Autodesk Inventor part; units mm, degrees
ref_plane "YZ Plane" through (0, 0, 0) normal (1, 0, 0) x (0, 1, 0)
ref_plane "XZ Plane" through (0, 0, 0) normal (0, 1, 0) x (-1, 0, 0)
ref_plane "XY Plane" through (0, 0, 0) normal (0, 0, 1) x (1, 0, 0)
sketch "Sketch1" plane through (0, 0, 0) normal (0, 1, 0) x (-1, 0, 0)
  arc A0 (-25.4, 0) -> (25.4, 0) centre (0, 0) ccw
  arc A1 (-35.4, 0) -> (35.4, 0) centre (0, 0) ccw
  line L0 (-35.4, 0) -> (-25.4, 0)
  line L1 (25.4, 0) -> (35.4, 0)
  line L2 (35.4, 0) -> (55.4, 0)
  line L3 (55.4, 0) -> (55.4, -10)
  line L4 (55.4, -10) -> (33.9582, -10)
  line L5 (-35.4, 0) -> (-55.4, 0)
  line L6 (-55.4, 0) -> (-55.4, -10)
  line L7 (-55.4, -10) -> (-33.9582, -10)
  dimension "d0" = 50.8
  dimension "d1" = 10
  dimension "d2" = 20
  dimension "d3" = 10
  dimension "d4" = 20
  dimension "d5" = 10
extrude "Extrusion1" add sketch "Sketch1" along normal blind 40
sketch "Sketch2" plane through (-55.4, 0, 0) normal (0, 0, 1) x (1, 0, 0)
  circle A0 centre (10, 20) radius 2.75
  circle A1 centre (100.8, 20) radius 2.75
  line L0 (80.8, 40) -> (110.8, 40)
  line L1 (110.8, 0) -> (110.8, 40)
  line L2 (0, 0) -> (0, 40)
  line L3 (0, 40) -> (30, 40)
  point P0 (55.4, 0)
  dimension "d8" = 5.5
  dimension "d9" = 5.5
  dimension "d10" = 20
  dimension "d11" = 10
  dimension "d12" = 10
  dimension "d13" = 20
extrude "Extrusion2" cut sketch "Sketch2" against normal blind 40
Source: CAD feature listing. Evaluate the final solid. Frame: model axes, mm. A direction names the side the tool comes from. Round coordinates to 2 decimals unless told otherwise and drop trailing zeros. Loops run counter-clockwise (first coordinate to the right, second up) from the corner with the lowest first, then second, coordinate; pieces in that order, holes last. Notation, with made-up numbers: (29, -17.75) -> (36, -17.75) arc R18 ccw to (36, 16.25) -> close; hole circle Ø9 at (61.25, 18.25). An arc over 180 degrees is marked (long way). Answer as a JSON object with one key per item and string values. Group by question number.
Q1. Contact query for flat-ended pins moving along their axis: P1, Ø3, axis at x = -9, y = 10.5, coming from the +Z side; P2, Ø6, axis at x = -19.5, z = -4, coming from the +Y side; P3, Ø4, axis at x = 7, y = 30.5, coming from the +Z side; P4, Ø10.5, axis at x = -41, y = 16.5, coming from the -Z side. Output: stop coordinate, or through.
Q2. Access query for faces 1 (the flat face through (1, 0, -29)), 2 (the flat face through (-42, 20, -10)), 3 (the flat face through (42, 20, -10)). Directions: +Z, -Z, +X, -X, +Y, -Y. A direction counts if a zero-diameter tool reaches every point of the face in a straight line with its end or side. Return the directions, or none.
Q3. Mould query, pull axis X, two halves, no side actions, for faces 4 (the cylindrical face through (-0.637, 19.72, -35.394)), 5 (the cylindrical face through (-48.147, 20.121, -4.93)), 6 (the flat face through (55.4, 20, -5)), 7 (the flat face through (41, 20, 0)). Classes: pulls with the +X half, pulls with the -X half, needs draft (parallel to the pull), parting line crosses it, or undercut.
Q4. Section query A-A (x = 45.4). Output: boundary loops of the cut face in (y, z), plus the area to 3 significant figures.
Q5. Section query B-B (y = 20). Output: boundary loops of the cut face in (x, z).
Q6. Section query C-C (z = -16.5). Output: boundary loops of the cut face in (x, y), plus the area to 3 significant figures.
Q7. Ray query, line 1 (Y direction, x = 45.4, z = -5); line 2 (X direction, y = 18, z = -9); line 3 (Z direction, x = 35.5, y = 18). Return the intervals inside material, ascending. Write a range as from..to.
Q8. Section query D-D (y = 8). Output: boundary loops of the cut face in (x, z).
Completed:
{
 "1": {"P1": "z = -23.13", "P2": "through", "P3": "z = -23.75", "P4": "z = -10"},
 "2": {"face 1": "+Z, -Z, +X, -X, -Y", "face 2": "-Z, -X, +Y, -Y", "face 3": "-Z, +X, +Y, -Y"},
 "3": {"face 4": "parting line crosses it", "face 5": "undercut", "face 6": "pulls with the +X half", "face 7": "needs draft"},
 "4": {"outline": "(0, -10) -> (17.25, -10) -> (17.25, 0) -> (0, 0) -> close; (22.75, -10) -> (40, -10) -> (40, 0) -> (22.75, 0) -> close", "area": "345 mm²"},
 "5": {"outline": "(-55.4, -10) -> (-48.15, -10) -> (-48.15, 0) -> (-55.4, 0) -> close; (-42.65, -10) -> (-33.96, -10) arc R35.4 ccw to (33.96, -10) -> (42.65, -10) -> (42.65, 0) -> (25.4, 0) arc R25.4 cw to (-25.4, 0) -> (-42.65, 0) -> close; (48.15, -10) -> (55.4, -10) -> (55.4, 0) -> (48.15, 0) -> close"},
 "6": {"outline": "(-31.32, 0) -> (-19.31, 0) -> (-19.31, 40) -> (-31.32, 40) -> close; (19.31, 0) -> (31.32, 0) -> (31.32, 40) -> (19.31, 40) -> close", "area": "961 mm²"},
 "7": {"line 1": "0..17.25, 22.75..40", "line 2": "-55.4..-47.29, -43.51..-23.75, 23.75..43.51, 47.29..55.4", "line 3": "-10..0"},
 "8": {"outline": "(-55.4, -10) -> (-33.96, -10) arc R35.4 ccw to (33.96, -10) -> (55.4, -10) -> (55.4, 0) -> (25.4, 0) arc R25.4 cw to (-25.4, 0) -> (-55.4, 0) -> close"}
}
